```python
from build123d import *

# Parameters (mm, degrees)
F1_DEPTH = 30
F3_DEPTH = 50.001
F5_DEPTH = 25
F6_DEPTH = 15


with BuildPart() as f1:
    # F0 (on Front) → F1 (new body)
    with BuildSketch(Plane.XZ):
        Polygon((0, 40), (0, 0), (50, 0), (50, 25), (25, 25), (10, 40), align=None)
    extrude(amount=F1_DEPTH)

    # F2 (on face) → F3 (cut, through all)
    with BuildSketch(Plane(origin=(0, 0, 0), x_dir=(0, -1, 0), z_dir=(-1, 0, 0))):
        Polygon((7.5, 40), (15, 31), (22.5, 40), align=None)
    extrude(amount=-F3_DEPTH, mode=Mode.SUBTRACT)

    # F4 (on face) → F5 (cut, through all)
    with BuildSketch(Plane.YZ.offset(50)):
        Polygon((-10, 20), (0, 25), (-30, 25), (-30, 10), (-20, 15), align=None)
    extrude(amount=-F5_DEPTH, mode=Mode.SUBTRACT)

    # F4 (on face) → F6 (cut)
    with BuildSketch(Plane.YZ.offset(50)):
        Polygon((-10, 0), (-10, 20), (-20, 15), (-20, 0), align=None)
    extrude(amount=-F6_DEPTH, mode=Mode.SUBTRACT)


solid = f1.part
```
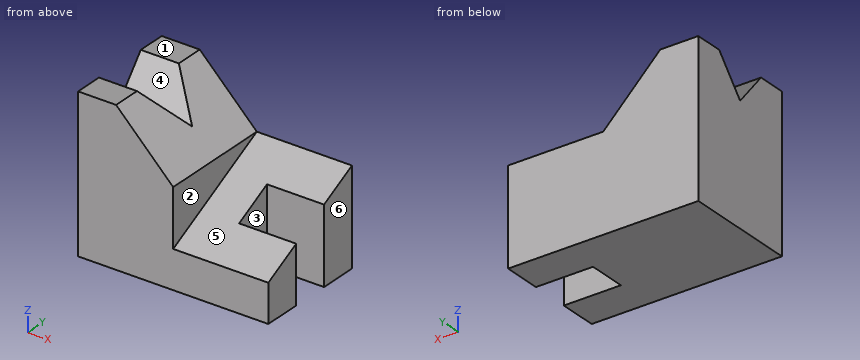
Design review of the part built by this model. Coordinates are the model's own, in mm. Face numbers are marked on the shaded views. A direction names the side the tool comes from. Coordinates: 2 decimals unless noted, no trailing zeros. Order: outer loops, then holes, each group sorted by start corner. A loop starts at its lowest first (then second) coordinate and runs counter-clockwise, first axis right, second up. Notation, with made-up numbers: (-0.75, 73) -> (57.25, 73) arc R12 cw to (57.25, 83) -> close; hole circle Ø9 at (33, -4). An arc over 180 degrees is marked (long way). One line per item, written item: value. Start each with the question number.
Q1. Take a section at D-D, the plane y = -6.5. State the section outline as (x, z) points.
Q2. Tool access review of the marked faces 1, 2 and 3: name each direction out of +Z, -Z, +X, -X, +Y, -Y from which nothing blocks a thin tool from reaching the whole face with its end or side.
Q3. For probe 1 along Y at (x, z) = (45.5, 2.5); probe 2 along X at (y, z) = (-14, 3.5); probe 3 along X at (y, z) = (-6.25, 35), list the stretches that pass through material, from the lowest coordinate up.
Q4. Mouldability with a two-part tool opening along Y and no side actions: class the marked faces 4, 5 and 6 as pulls with the +Y half, pulls with the -Y half, needs draft (parallel to the pull), parting line crosses it, or undercut.
Q5. Take a section at A-A, the plane z = 13. State the section outline as (x, y) points, then the cut area to 3 significant figures.
Q6. Insertion check: pin 1 Ø1.5 at (x, y) = (23.5, -17) entering from +Z; pin 2 Ø1.5 at (x, z) = (33.5, 19) entering from -Y; pin 3 Ø6 at (y, z) = (-6, 27.5) entering from +X. Each pin has a flat end and moves straight along its axis. Give the tip position at first contact, or say it passes through.
Q7. Take a section at C-C, the plane z = 32.5. State the section outline as (x, y) points.
Q8. Take a section at B-B, the plane x = 37. State the section outline as (y, z) points, then the cut area to 3 significant figures.
Values follow:
1. outline: (0, 0) -> (50, 0) -> (50, 21.75) -> (25, 21.75) -> (25, 25) -> (10, 40) -> (0, 40) -> close
2. face 1: +Z, +X, -X, +Y, -Y
2. face 2: +Z, +X, -Y
2. face 3: +Z, -Z, +X
3. probe 1: y = -30 to -20, -10 to 0
3. probe 2: x = 0 to 35
3. probe 3: x = 0 to 15
4. face 4: undercut
4. face 5: pulls with the -Y half
4. face 6: needs draft
5. outline: (0, -30) -> (25, -30) -> (25, -24) -> (50, -24) -> (50, -20) -> (35, -20) -> (35, -10) -> (50, -10) -> (50, 0) -> (0, 0) -> close
5. area: 1,200 mm2
6. pin 1: stops at z = 27.25
6. pin 2: stops at y = -13.5
6. pin 3: stops at x = 25
7. outline: (0, -30) -> (17.5, -30) -> (17.5, -16.25) -> (0, -16.25) -> close; (0, -13.75) -> (17.5, -13.75) -> (17.5, 0) -> (0, 0) -> close
8. outline: (-30, 0) -> (-20, 0) -> (-20, 15) -> (-30, 10) -> close; (-10, 0) -> (0, 0) -> (0, 25) -> (-10, 20) -> close
8. area: 350 mm2
